Build history of the part. All positions in model axes, mm. Face numbers are marked on the shaded views. Round coordinates to 2 decimals unless told otherwise and drop trailing zeros. Write each loop counter-clockwise with the first axis right and the second up, starting at its lowest first coordinate (ties: lowest second). Pieces come first, ordered by that corner, then holes. Notation, with made-up numbers: M 53,6 L 63,6 A35 cw 63,38 Z; hole C 6,29 d7. An arc over 180 degrees is marked long. One line per item, written item: value. Start each with the question number.
```python
from build123d import *

# Parameters (mm, degrees)
SKETCH1_R           = 17.5
BOSS_EXTRUDE1_DEPTH = 1
SKETCH3_R           = 3
BOSS_EXTRUDE2_DEPTH = 10
FILLET1_R           = 2
SKETCH4_R           = 2
CUT_EXTRUDE1_DEPTH  = 7
BOSS_EXTRUDE3_START = 140
SKETCH5_R           = 2
BOSS_EXTRUDE3_DEPTH = 140
SKETCH6_R           = 3.5
BOSS_EXTRUDE4_DEPTH = 14
SKETCH8_R           = 7.5
BOSS_EXTRUDE5_DEPTH = 12
BOSS_EXTRUDE6_DEPTH = 2


with BuildPart() as part:
    # Sketch1 → Boss-Extrude1 (new body)
    with BuildSketch(Plane.XY):
        Circle(SKETCH1_R)
    extrude(amount=BOSS_EXTRUDE1_DEPTH)

    # Sketch3 → Boss-Extrude2 (add)
    with BuildSketch(Plane.XY.offset(1)):
        Circle(SKETCH3_R)
    extrude(amount=BOSS_EXTRUDE2_DEPTH)

    # Loft1: read off the stored shape, not the designer's step
    # Loft1: loft between two sections, ruled curve by curve
    loft1_from = [
        Edge.make_bspline([(1.044538227, -2.81228375, 11), (-4.580029274, -4.901360204, 11), (-6.669105728, 0.723207296, 11), (-1.044538227, 2.81228375, 11), (4.580029274, 4.901360204, 11), (6.669105728, -0.723207296, 11), (1.044538227, -2.81228375, 11)], [0, 0, 0, 0, 0.5, 0.5, 0.5, 1, 1, 1, 1], 3, [1, 0.333333333, 0.333333333, 1, 0.333333333, 0.333333333, 1]),
    ]
    loft1_to = [
        Edge.make_bspline([(5.441388928, -5.161519789, 1), (-4.88165065, -16.044297645, 1), (-15.764428506, -5.721258067, 1), (-5.441388928, 5.161519789, 1), (4.88165065, 16.044297645, 1), (15.764428506, 5.721258067, 1), (5.441388928, -5.161519789, 1)], [0, 0, 0, 0, 0.5, 0.5, 0.5, 1, 1, 1, 1], 3, [1, 0.333333333, 0.333333333, 1, 0.333333333, 0.333333333, 1]),
    ]
    loft1 = Solid(Shell([*[Face.make_surface_from_curves(loft1_from[k], loft1_to[k]) for k in range(1)], Face(Wire(loft1_from)), Face(Wire(loft1_to))]))
    add(loft1)

    # Fillet1
    fillet1_edges = [part.edges().sort_by_distance(p)[0] for p in [
        (-5.441388928, 5.161519789, 1),
    ]]
    fillet(fillet1_edges, radius=FILLET1_R)

    # Sketch4 → Cut-Extrude1 (cut)
    with BuildSketch(Plane.XY.offset(11)):
        Circle(SKETCH4_R)
    extrude(amount=-CUT_EXTRUDE1_DEPTH, mode=Mode.SUBTRACT)

    # Sketch5 → Boss-Extrude3 (add)
    with BuildSketch(Plane.XY.offset(4).offset(BOSS_EXTRUDE3_START)):
        Circle(SKETCH5_R)
    extrude(amount=-BOSS_EXTRUDE3_DEPTH)

    # Sketch6 → Boss-Extrude4 (add)
    with BuildSketch(Plane.XY.offset(144)):
        Circle(SKETCH6_R)
    extrude(amount=-BOSS_EXTRUDE4_DEPTH)

    # Loft2: read off the stored shape, not the designer's step
    # Loft2: loft between two sections, ruled curve by curve
    loft2_from = [
        Edge.make_bspline([(2.496146584, -7.072429019, 144), (-11.648711454, -12.064722187, 144), (-16.641004622, 2.080135851, 144), (-2.496146584, 7.072429019, 144), (11.648711454, 12.064722187, 144), (16.641004622, -2.080135851, 144), (2.496146584, -7.072429019, 144)], [0, 0, 0, 0, 0.5, 0.5, 0.5, 1, 1, 1, 1], 3, [1, 0.333333333, 0.333333333, 1, 0.333333333, 0.333333333, 1]),
    ]
    loft2_to = [
        Edge.make_bspline([(0.28118335, -3.488686848, 130), (-6.696190346, -4.051053549, 130), (-7.258557046, 2.926320147, 130), (-0.28118335, 3.488686848, 130), (6.696190346, 4.051053549, 130), (7.258557046, -2.926320147, 130), (0.28118335, -3.488686848, 130)], [0, 0, 0, 0, 0.5, 0.5, 0.5, 1, 1, 1, 1], 3, [1, 0.333333333, 0.333333333, 1, 0.333333333, 0.333333333, 1]),
    ]
    loft2 = Solid(Shell([*[Face.make_surface_from_curves(loft2_from[k], loft2_to[k]) for k in range(1)], Face(Wire(loft2_from)), Face(Wire(loft2_to))]))
    add(loft2)

    # Sketch8 → Boss-Extrude5 (add)
    with BuildSketch(Plane.XY.offset(144)):
        with Locations(Location((0, 0, 0), (0, 0, 289.44))):
            Circle(SKETCH8_R)
    extrude(amount=BOSS_EXTRUDE5_DEPTH)

    # Sketch9 → Boss-Extrude6 (add)
    with BuildSketch(Plane.XY.offset(156)):
        with BuildLine():
            Line((-18, 3), (-10.908712115, 3))
            ThreePointArc((-10.908712115, 3), (-9.828588665, 3.316749177), (-9.090593429, 4.166666667))
            ThreePointArc((-9.090593429, 4.166666667), (-7.071067812, 7.071067812), (-4.166666667, 9.090593429))
            ThreePointArc((-4.166666667, 9.090593429), (-3.316749177, 9.828588665), (-3, 10.908712115))
            Line((-3, 10.908712115), (-3, 18))
            ThreePointArc((-3, 18), (-2.414213562, 19.414213562), (-1, 20))
            Line((-1, 20), (1, 20))
            ThreePointArc((1, 20), (2.414213562, 19.414213562), (3, 18))
            Line((3, 18), (3, 10.908712115))
            ThreePointArc((3, 10.908712115), (3.316749177, 9.828588665), (4.166666667, 9.090593429))
            ThreePointArc((4.166666667, 9.090593429), (7.071067812, 7.071067812), (9.090593429, 4.166666667))
            ThreePointArc((9.090593429, 4.166666667), (9.828588665, 3.316749177), (10.908712115, 3))
            Line((10.908712115, 3), (18, 3))
            ThreePointArc((18, 3), (19.414213562, 2.414213562), (20, 1))
            Line((20, 1), (20, -1))
            ThreePointArc((20, -1), (19.414213562, -2.414213562), (18, -3))
            Line((18, -3), (10.908712115, -3))
            ThreePointArc((10.908712115, -3), (9.828588665, -3.316749177), (9.090593429, -4.166666667))
            ThreePointArc((9.090593429, -4.166666667), (7.071067812, -7.071067812), (4.166666667, -9.090593429))
            ThreePointArc((4.166666667, -9.090593429), (3.316749177, -9.828588665), (3, -10.908712115))
            Line((3, -10.908712115), (3, -18))
            ThreePointArc((3, -18), (2.414213562, -19.414213562), (1, -20))
            Line((1, -20), (-1, -20))
            ThreePointArc((-1, -20), (-2.414213562, -19.414213562), (-3, -18))
            Line((-3, -18), (-3, -10.908712115))
            ThreePointArc((-3, -10.908712115), (-3.316749177, -9.828588665), (-4.166666667, -9.090593429))
            ThreePointArc((-4.166666667, -9.090593429), (-7.071067812, -7.071067812), (-9.090593429, -4.166666667))
            ThreePointArc((-9.090593429, -4.166666667), (-9.828588665, -3.316749177), (-10.908712115, -3))
            Line((-10.908712115, -3), (-18, -3))
            ThreePointArc((-18, -3), (-19.414213562, -2.414213562), (-20, -1))
            Line((-20, -1), (-20, 1))
            ThreePointArc((-20, 1), (-19.414213562, 2.414213562), (-18, 3))
        make_face()
        with BuildLine():
            Line((-17.145168387, 1.019387686), (-10, 1.019387686))
            ThreePointArc((-10, 1.019387686), (-8.980612314, 0), (-10, -1.019387686))
            Line((-10, -1.019387686), (-17.145168387, -1.019387686))
            ThreePointArc((-17.145168387, -1.019387686), (-18.164556073, 0), (-17.145168387, 1.019387686))
        make_face(mode=Mode.SUBTRACT)
        with BuildLine():
            Line((-1.019387686, 17.145168387), (-1.019387686, 10))
            ThreePointArc((-1.019387686, 10), (0, 8.980612314), (1.019387686, 10))
            Line((1.019387686, 10), (1.019387686, 17.145168387))
            ThreePointArc((1.019387686, 17.145168387), (0, 18.164556073), (-1.019387686, 17.145168387))
        make_face(mode=Mode.SUBTRACT)
        with BuildLine():
            Line((1.019387686, -17.145168387), (1.019387686, -10))
            ThreePointArc((1.019387686, -10), (0, -8.980612314), (-1.019387686, -10))
            Line((-1.019387686, -10), (-1.019387686, -17.145168387))
            ThreePointArc((-1.019387686, -17.145168387), (0, -18.164556073), (1.019387686, -17.145168387))
        make_face(mode=Mode.SUBTRACT)
        with BuildLine():
            Line((17.145168387, -1.019387686), (10, -1.019387686))
            ThreePointArc((10, -1.019387686), (8.980612314, 0), (10, 1.019387686))
            Line((10, 1.019387686), (17.145168387, 1.019387686))
            ThreePointArc((17.145168387, 1.019387686), (18.164556073, 0), (17.145168387, -1.019387686))
        make_face(mode=Mode.SUBTRACT)
    extrude(amount=BOSS_EXTRUDE6_DEPTH)


solid = part.part
```
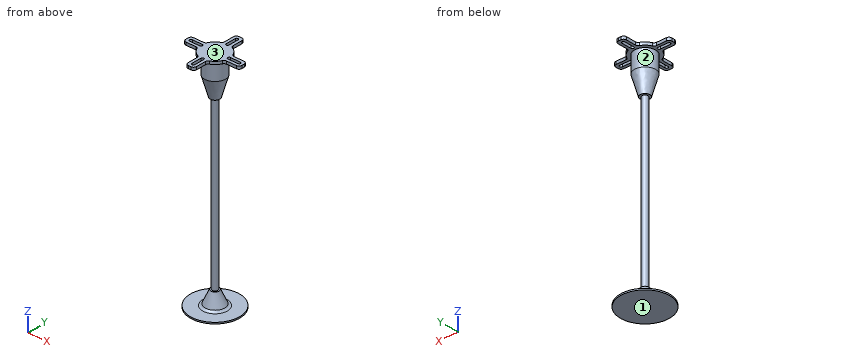
Item 1: Two-plate mould, pull along Z, no slides. Class the marked faces 1, 2 and 3: pulls with the +Z half, pulls with the -Z half, needs draft (parallel to the pull), parting line crosses it, or undercut.
Item 2: Drill centre lines: line 1 (Z direction, x = 7, y = 5.5); line 2 (Z direction, x = 11, y = 8); line 3 (Y direction, x = 0, z = 104). Where is each one in solid material? Low to high.
Item 3: Cut at A-A, the plane z = 91.5. Write the cut outline in (x, y), plus the area to 3 significant figures.
Item 4: Drop flat-ended pins along their axis: pin 1 (1.6 mm diameter, centred on x = -13, z = 157, fed in from -Y); pin 2 (1.6 mm diameter, centred on y = 13, z = 157, fed in from -X); pin 3 (6 mm diameter, centred on y = -7.5, z = 79, fed in from -X); pin 4 (1 mm diameter, centred on x = -12, z = 157, fed in from +Y). Give the stop position or say it passes through.
Computed values:
1. face 1: pulls with the -Z half
1. face 2: undercut
1. face 3: pulls with the +Z half
2. line 1: z = 0 to 1, 156 to 158
2. line 2: z = 0 to 1
2. line 3: y = -2 to 2
3. outline: C 0,0 d4
3. area: 12.6 mm2
4. pin 1: stops at y = -3
4. pin 2: stops at x = -3
4. pin 3: passes through
4. pin 4: stops at y = 3
